The listing builds one solid part. Answer for the finished solid, in the listing's coordinates (mm). A direction names the side the tool comes from. Round coordinates to 2 decimals unless told otherwise and drop trailing zeros. Write each loop counter-clockwise with the first axis right and the second up, starting at its lowest first coordinate (ties: lowest second). Pieces come first, ordered by that corner, then holes. Notation, with made-up numbers: (-26.75, 57.25) - (-2.75, 57.25) arc R24 cw to (-2.75, 81.25) - close; hole circle Ø6 at (7, 47). An arc over 180 degrees is marked (long way). Return JSON: item names as keys, results as strings. Group by question number.
Autodesk Inventor part; units mm, degrees
ref_plane "Work Plane1" through (0, 0, 279.4) normal (0, 0, 1) x (1, 0, 0)
ref_plane "YZ Plane" through (0, 0, 0) normal (1, 0, 0) x (0, 1, 0)
ref_plane "XZ Plane" through (0, 0, 0) normal (0, 1, 0) x (-1, 0, 0)
sketch "Sketch1" plane through (0, 0, 0) normal (0, 0, 1) x (1, 0, 0)
  circle A0 centre (0, 0) radius 50.8
  dimension "d0" = 101.6
ref_plane "Work Plane1" through (0, 0, 279.4) normal (0, 0, 1) x (1, 0, 0)
sketch "Sketch2" plane through (0, 0, 279.4) normal (0, 0, 1) x (1, 0, 0)
  circle A0 centre (0, 0) radius 7.1437
  dimension "d3" = 14.2875
loft "Loft2" add profiles "Sketch1", "Sketch2"
sketch "Sketch15" plane through (0, 0, 0) normal (0, 1, 0) x (-1, 0, 0)
  line L0 (-7.1437, 279.4) -> (7.1437, 279.4)
  line L1 (0, 279.4) -> (-7.1437, 279.4)
  line L2 (-50.8, 0) -> (50.8, 0)
  line L3 (50.8, 0) -> (-50.8, 0)
  line L4 (-50.8, 0) -> (-50.8, 279.4)
  line L5 (-50.8, 279.4) -> (50.8, 279.4)
  line L6 (50.8, 279.4) -> (50.8, 0)
  line L7 (-7.1437, 279.4) -> (0, 302.26)
  line L8 (0, 279.4) -> (0, 88.9)
  line L9 (0, 88.9) -> (-46.3803, 88.9)
  line L10 (0, 0) -> (-50.8, 0)
  line L11 (0, 88.9) -> (0, 0)
  line L12 (0, 84.1375) -> (-46.8411, 84.1375)
  line L13 (0, 68.2625) -> (-48.1941, 68.2625)
  line L14 (-48.1941, 68.2625) -> (-45.0191, 68.2625)
  line L15 (-45.0191, 68.2625) -> (-45.0191, 65.0875)
  line L16 (-45.0191, 65.0875) -> (-45.2731, 65.0875)
  line L17 (-45.2731, 65.0875) -> (-45.0191, 68.2625)
  line L18 (-45.2731, 65.0875) -> (0, 65.0875)
  point P0 (0, 0)
  dimension "d258" = 190.5
  dimension "d259" = 88.9
  dimension "d264" = 4.7625
  dimension "d315" = 3.175
  dimension "d316" = 3.175
  dimension "d317" = 0.254
  dimension "d330" = 15.875
extrude "Extrusion37" cut sketch "Sketch15" along normal through all both and the other way through all
revolve "Revolution11" add sketch "Sketch15" angle 360 about axis through (0, 0, 88.9) along (0, 0, -1) contours L11 L18 L15 L13 | L15 L16 L17
sketch "Sketch59" plane through (0, 0, 68.2625) normal (0, 0, 1) x (1, 0, 0)
  line L0 (0, 0) -> (0, 41.91)
  circle A0 centre (0, 41.91) radius 5.334
  circle A1 centre (-36.2951, 20.955) radius 5.334
  circle A2 centre (-36.2951, -20.955) radius 5.334
  circle A3 centre (0, -41.91) radius 5.334
  circle A4 centre (36.2951, -20.955) radius 5.334
  circle A5 centre (36.2951, 20.955) radius 5.334
  dimension "d319" = 41.91
  dimension "d320" = 10.668
  dimension "d323" = 360
extrude "Extrusion45" cut sketch "Sketch59" against normal blind 25.4
sketch "Sketch60" plane through (0, -41.91, 65.0875) normal (0, 0, -1) x (-1, 0, 0)
  circle A0 centre (0, 41.91) radius 17.5
  point P0 (0, 41.91)
  dimension "d327" = 35
extrude "Extrusion46" cut sketch "Sketch60" against normal blind 25.4
sketch "Sketch61" plane through (0, -41.91, 65.0875) normal (0, 0, -1) x (-1, 0, 0)
  line L0 (18, 45.085) -> (37.05, 45.085)
  line L1 (37.05, 45.085) -> (37.05, 35.56)
  line L2 (37.05, 35.56) -> (18, 35.56)
  line L3 (18, 35.56) -> (18, 45.085)
  line L4 (0, 41.91) -> (0, -3.2701)
  line L5 (-18, 45.085) -> (-37.05, 45.085)
  line L6 (-37.05, 45.085) -> (-37.05, 35.56)
  line L7 (-37.05, 35.56) -> (-18, 35.56)
  line L8 (-18, 35.56) -> (-18, 45.085)
  dimension "d331" = 19.05
  dimension "d332" = 9.525
  dimension "d333" = 18
  dimension "d347" = 3.175
extrude "Extrusion47" add sketch "Sketch61" along normal blind 6.604
sketch "Sketch62" plane through (18, 3.175, 65.0875) normal (0, 1, 0) x (1, 0, 0)
  line L0 (-23.334, 0) -> (-12.666, 0)
  line L1 (-18, 0) -> (-18, 51.1143)
  line L2 (19.05, 0) -> (0, 0)
  line L3 (19.05, 0) -> (19.05, 6.604)
  line L4 (0, 6.604) -> (19.05, 6.604)
  line L5 (0, 0) -> (0, 6.604)
  circle A0 centre (14.605, 2.794) radius 1.27
  circle A1 centre (4.445, 2.794) radius 1.27
  line L6 (19.05, 6.604) -> (0, 6.604)
  line L7 (9.525, 6.604) -> (9.525, 11.5709)
  circle A2 centre (-50.605, 2.794) radius 1.27
  circle A3 centre (-40.445, 2.794) radius 1.27
  point P0 (-18, 65.0875)
  point P1 (-22.2982, 0)
  point P2 (-13.7018, 0)
  dimension "d337" = 2.54
  dimension "d338" = 2.54
  dimension "d339" = 10.16
  dimension "d342" = 5.08
  dimension "d345" = 3.81
  dimension "d346" = 3.81
extrude "Extrusion48" cut sketch "Sketch62" against normal through all contours A0 | A1 | A2 | A3
properties part number "aftServoAssemblyForwardDisc"
(1) Determine the mould class of faces 1 (the cylindrical face through (13.887, -10.648, 66.653)), 2 (the cylindrical face through (-32.02, -1.52, 63.42)), 3 (the conical face through (-45.147, -0.271, 66.653)), 4 (the cylindrical face through (-22.72, -1.521, 63.533)) for opening direction Z: +Z half, -Z half, draft (parallel to the pull), parting line (faces both ways), or undercut.
(2) For faces 5 (the flat face through (-27, 3.175, 62)), 6 (the cylindrical face through (-31.76, 18.15, 66.7)), 7 (the flat face through (-37.05, -2, 62)), determine the directions among +Z, -Z, +X, -X, +Y, -Y from which every point of the face is accessible in a straight line to the end or side of a thin tool.
(3) Find section A-A (x = 0). Write down the section's boundary in (y, z), plus the area to 3 significant figures.
(4) Find section B-B (y = 0). State how many separate pieces and enclosed holes the cut face has, plus the area to 3 significant figures.
(5) Consider line 1 (Y direction, x = 0, z = 67.6); line 2 (Z direction, x = 13.5, y = -32.5); line 3 (Y direction, x = 34, z = 67.5). Determine where each line is inside the solid, lowest interval first.
(6) Flat-ended cylindrical pins translate along their axes: pin 1 (5 mm diameter, centred on y = 0, z = 61.5, fed in from -X); pin 2 (1.5 mm diameter, centred on x = 22.44, z = 62.29, fed in from -Y); pin 3 (4 mm diameter, centred on x = 32.6, z = 62.29, fed in from -Y); pin 4 (17 mm diameter, centred on x = 0, y = 41.91, fed in from -Z). Find the tip coordinate at first contact, or state that the pin passes through.
(7) Find section C-C (z = 66.25). Write down the section's boundary in (x, y) (3 decimals).
Check sheet entries:
{
 "1": {"face 1": "draft", "face 2": "undercut", "face 3": "+Z half", "face 4": "undercut"},
 "2": {"face 5": "-Z, +X, -X, +Y", "face 6": "+Z, -Z", "face 7": "-Z, -X, +Y, -Y"},
 "3": {"outline": "(-36.58, 65.09) - (-17.5, 65.09) - (-17.5, 68.26) - (-36.58, 68.26) - close; (17.5, 65.09) - (36.58, 65.09) - (36.58, 68.26) - (17.5, 68.26) - close", "area": "121 mm^2"},
 "4": {"separate pieces": "2", "enclosed holes": "4", "area": "407 mm^2"},
 "5": {"line 1": "y = -36.58 to -17.5, 17.5 to 36.58", "line 2": "z = 65.09 to 68.26", "line 3": "y = -29.6 to -25.77, -16.14 to 16.14, 25.77 to 29.6"},
 "6": {"pin 1": "stops at x = -37.05", "pin 2": "passes through", "pin 3": "stops at y = -6.35", "pin 4": "stops at z = 65.09"},
 "7": {"outline": "(-41.129, -18.699) arc R5.334 cw (long way) to (-36.759, -26.269) arc R45.18 ccw to (-4.37, -44.968) arc R5.334 cw (long way) to (4.37, -44.968) arc R45.18 ccw to (36.759, -26.269) arc R5.334 cw (long way) to (41.129, -18.699) arc R45.18 ccw to (41.129, 18.699) arc R5.334 cw (long way) to (36.759, 26.269) arc R45.18 ccw to (4.37, 44.968) arc R5.334 cw (long way) to (-4.37, 44.968) arc R45.18 ccw to (-36.759, 26.269) arc R5.334 cw (long way) to (-41.129, 18.699) arc R45.18 ccw to start; hole circle Ø35 at (0, 0)"}
}
